```python
from build123d import *

# Parameters (mm, degrees)
F0_R     = 2
F1_DEPTH = 1
F2_R     = 0.99999


# Not quite as in the source:
# - a fillet or chamfer is up to 0.001 mm smaller than in the source, because OpenCascade refuses the exact size


with BuildPart() as f1:
    # F0 (on Top) → F1 (new body)
    with BuildSketch(Plane.XY):
        with BuildLine():
            Line((-56.070427214, 21.7097375971), (-58.2998616904, 23.7171294162))
            Line((-58.2998616904, 23.7171294162), (-61.9800800254, 19.6298328761))
            ThreePointArc((-61.9800800254, 19.6298328761), (-63.5129882811, 15.3010335004), (-61.5359947107, 11.156180285))
            Line((-61.5359947107, 11.156180285), (-35.2268663082, -12.5326653305))
            ThreePointArc((-35.2268663082, -12.5326653305), (-31.2120826701, -14.0737963776), (-27.1972990319, -12.5326653305))
            Line((-27.1972990319, -12.5326653305), (0, 11.9558927118))
            Line((0, 11.9558927118), (27.1972990319, -12.5326653305))
            ThreePointArc((27.1972990319, -12.5326653305), (31.2120826701, -14.0737963776), (35.2268663082, -12.5326653305))
            Line((35.2268663082, -12.5326653305), (61.5359947107, 11.156180285))
            ThreePointArc((61.5359947107, 11.156180285), (63.5129882811, 15.3010335004), (61.9800800254, 19.6298328761))
            Line((61.9800800254, 19.6298328761), (58.2998616904, 23.7171294162))
            Line((58.2998616904, 23.7171294162), (56.070427214, 21.7097375971))
            Line((56.070427214, 21.7097375971), (33.7760824497, 1.6358194063))
            Line((33.7760824497, 1.6358194063), (31.2120826701, -0.6728163648))
            Line((31.2120826701, -0.6728163648), (28.6480828904, 1.6358194063))
            Line((28.6480828904, 1.6358194063), (1.8948691733, 25.7245212353))
            Line((1.8948691733, 25.7245212353), (0, 27.4306691023))
            Line((0, 27.4306691023), (-1.8948691733, 25.7245212353))
            Line((-1.8948691733, 25.7245212353), (-28.6480828904, 1.6358194063))
            Line((-28.6480828904, 1.6358194063), (-31.2120826701, -0.6728163648))
            Line((-31.2120826701, -0.6728163648), (-33.7760824497, 1.6358194063))
            Line((-33.7760824497, 1.6358194063), (-56.070427214, 21.7097375971))
        make_face()
        with Locations((-31.2120826701, -8.0737963776)):
            Circle(F0_R, mode=Mode.SUBTRACT)
        Polygon((-53.6574585069, 9.4448453424), (-50.9809360815, 12.4174246443), (-35.0758352357, -1.9035924822), (-37.7523576611, -4.8761717841), align=None, mode=Mode.SUBTRACT)
        Polygon((-6.0931870421, 11.8520933749), (-22.4423732026, -2.868779965), (-25.118895628, 0.1037993369), (-8.7697094675, 14.8246726768), align=None, mode=Mode.SUBTRACT)
        with Locations((31.2120826701, -8.0737963776)):
            Circle(F0_R, mode=Mode.SUBTRACT)
        Polygon((22.4423732026, -2.868779965), (6.0931870421, 11.8520933749), (8.7697094675, 14.8246726768), (25.118895628, 0.1037993369), align=None, mode=Mode.SUBTRACT)
        Polygon((37.7523576611, -4.8761717841), (35.0758352357, -1.9035924822), (51.0113683193, 12.4448259544), (53.6878907447, 9.4722466525), align=None, mode=Mode.SUBTRACT)
        with Locations((-57.5212110725, 15.6150492379)):
            Circle(F0_R, mode=Mode.SUBTRACT)
        with Locations((0, 20.0296890894)):
            Circle(F0_R, mode=Mode.SUBTRACT)
        with Locations((57.5516433104, 15.6424505479)):
            Circle(F0_R, mode=Mode.SUBTRACT)
        Polygon((-55.7358619108, 22.0813100098), (-57.9652963872, 24.0887018289), (-58.2998616904, 23.7171294162), (-56.070427214, 21.7097375971), align=None)
        Polygon((-57.6307310841, 24.4602742417), (-57.9652963872, 24.0887018289), (-55.7358619108, 22.0813100098), (-55.4012966076, 22.4528824226), align=None)
        with BuildLine():
            Line((-53.9505127491, 28.5475707818), (-57.6307310841, 24.4602742417))
            Line((-57.6307310841, 24.4602742417), (-55.4012966076, 22.4528824226))
            Line((-55.4012966076, 22.4528824226), (-33.1069518433, 2.3789642318))
            Line((-33.1069518433, 2.3789642318), (-31.2120826701, 0.6728163648))
            Line((-31.2120826701, 0.6728163648), (-29.3172134968, 2.3789642318))
            Line((-29.3172134968, 2.3789642318), (-2.5639997796, 26.4676660607))
            Line((-2.5639997796, 26.4676660607), (0, 28.7763018319))
            Line((0, 28.7763018319), (2.5639997796, 26.4676660607))
            Line((2.5639997796, 26.4676660607), (29.3172134968, 2.3789642318))
            Line((29.3172134968, 2.3789642318), (31.2120826701, 0.6728163648))
            Line((31.2120826701, 0.6728163648), (33.1069518433, 2.3789642318))
            Line((33.1069518433, 2.3789642318), (55.4012966076, 22.4528824226))
            Line((55.4012966076, 22.4528824226), (57.6307310841, 24.4602742417))
            Line((57.6307310841, 24.4602742417), (53.9505127491, 28.5475707818))
            ThreePointArc((53.9505127491, 28.5475707818), (49.8056595337, 30.5245643522), (45.4768601581, 28.9916560965))
            Line((45.4768601581, 28.9916560965), (31.2120826701, 16.1475927553))
            Line((31.2120826701, 16.1475927553), (4.0147836382, 40.6361507976))
            ThreePointArc((4.0147836382, 40.6361507976), (0, 42.1772818447), (-4.0147836382, 40.6361507976))
            Line((-4.0147836382, 40.6361507976), (-31.2120826701, 16.1475927553))
            Line((-31.2120826701, 16.1475927553), (-45.4768601581, 28.9916560965))
            ThreePointArc((-45.4768601581, 28.9916560965), (-49.8056595337, 30.5245643522), (-53.9505127491, 28.5475707818))
        make_face()
        with Locations((-31.2120826701, 8.0737963776)):
            Circle(F0_R, mode=Mode.SUBTRACT)
        with Locations((31.2120826701, 8.0737963776)):
            Circle(F0_R, mode=Mode.SUBTRACT)
        Polygon((-46.3710360561, 19.0317138545), (-43.6945136306, 22.0042931564), (-34.3115040691, 13.5557933995), (-37.0313460748, 10.6222192229), align=None, mode=Mode.SUBTRACT)
        with Locations((-49.4916437962, 24.5327871436)):
            Circle(F0_R, mode=Mode.SUBTRACT)
        Polygon((-22.4423732026, 13.2788127903), (-25.118895628, 16.2513920922), (-8.7697094675, 30.9722654321), (-6.0931870421, 27.9996861302), align=None, mode=Mode.SUBTRACT)
        Polygon((6.0931870421, 27.9996861302), (8.7697094675, 30.9722654321), (25.118895628, 16.2513920922), (22.4423732026, 13.2788127903), align=None, mode=Mode.SUBTRACT)
        Polygon((37.0092128356, 10.6022903648), (34.3326904102, 13.5748696667), (43.6361429708, 21.9517359782), (46.3126653962, 18.9791566763), align=None, mode=Mode.SUBTRACT)
        with Locations((49.4332731364, 24.4802299654)):
            Circle(F0_R, mode=Mode.SUBTRACT)
        with Locations((0, 36.1772818447)):
            Circle(F0_R, mode=Mode.SUBTRACT)
        Polygon((-31.2120826701, 0), (-33.4415171465, 2.0073918191), (-33.7760824497, 1.6358194063), (-31.2120826701, -0.6728163648), (-28.6480828904, 1.6358194063), (-28.9826481936, 2.0073918191), align=None)
        Polygon((-33.1069518433, 2.3789642318), (-33.4415171465, 2.0073918191), (-31.2120826701, 0), (-28.9826481936, 2.0073918191), (-29.3172134968, 2.3789642318), (-31.2120826701, 0.6728163648), align=None)
        Polygon((0, 28.1034854671), (-2.2294344764, 26.096093648), (-1.8948691733, 25.7245212353), (0, 27.4306691023), (1.8948691733, 25.7245212353), (2.2294344764, 26.096093648), align=None)
        Polygon((-2.5639997796, 26.4676660607), (-2.2294344764, 26.096093648), (0, 28.1034854671), (2.2294344764, 26.096093648), (2.5639997796, 26.4676660607), (0, 28.7763018319), align=None)
        Polygon((31.2120826701, 0), (28.9826481936, 2.0073918191), (28.6480828904, 1.6358194063), (31.2120826701, -0.6728163648), (33.7760824497, 1.6358194063), (33.4415171465, 2.0073918191), align=None)
        Polygon((29.3172134968, 2.3789642318), (28.9826481936, 2.0073918191), (31.2120826701, 0), (33.4415171465, 2.0073918191), (33.1069518433, 2.3789642318), (31.2120826701, 0.6728163648), align=None)
        Polygon((57.9652963872, 24.0887018289), (55.7358619108, 22.0813100098), (56.070427214, 21.7097375971), (58.2998616904, 23.7171294162), align=None)
        Polygon((57.9652963872, 24.0887018289), (57.6307310841, 24.4602742417), (55.4012966076, 22.4528824226), (55.7358619108, 22.0813100098), align=None)
    extrude(amount=F1_DEPTH)

    # F2 (radius 1 in the source; OpenCascade refuses exactly that, so slightly less here)
    f2_edges = [f1.edges().sort_by_distance(p)[0] for p in [
        (-63.512988, 15.301034, 1),
        (-48.381431, -0.688243, 1),
        (-31.212083, -14.073796, 1),
        (-13.59865, -0.288386, 1),
        (13.59865, -0.288386, 1),
        (31.212083, -14.073796, 1),
        (48.381431, -0.688243, 1),
        (63.512988, 15.301034, 1),
        (57.965296, 24.088702, 1),
        (49.80566, 30.524564, 1),
        (38.344471, 22.569624, 1),
        (17.613433, 28.391872, 1),
        (0, 42.177282, 1),
        (-17.613433, 28.391872, 1),
        (-38.344471, 22.569624, 1),
        (-49.80566, 30.524564, 1),
        (-57.965296, 24.088702, 1),
    ]]
    fillet(f2_edges, radius=F2_R)


solid = f1.part
```
Input: part model. Units: mm. Frame: model coordinates. Coordinates: 2 decimals unless noted, no trailing zeros. Put each result on its own line as item: value. Start each with the question number.
1) Mould query, pull axis Y, two halves, no side actions, for faces 1 (the face through (-51.08, 23.32, 0.49)), 2 (the face through (-45.59, 2.18, 0.49)), 3 (the face through (48.375, -0.311, 0.699)). Classes: pulls with the +Y half, pulls with the -Y half, needs draft (parallel to the pull), parting line crosses it, or undercut.
2) Contact query for a flat-ended pin moving along its axis: pin 1 (2.5 mm diameter, centred on x = 57.55, y = 15.64, fed in from -Z). Output: stop coordinate, or through.
3) Ray query, L1, parallel to Y at x = 51, z = 0.4; L2, parallel to Y at x = 29.5, z = 0.45; L3, parallel to Y at x = 35, z = 0.15. Return the intervals inside material, ascending.
4) Cut plane A-A (x = 11.5). State how many separate pieces and enclosed holes the cut face has, plus the area to 3 significant figures.
Resolved:
1. face 1: undercut
1. face 2: undercut
1. face 3: pulls with the -Y half
2. pin 1: passes through
3. L1: y = 1.78 to 7.05, 12.43 to 17.14, 18.49 to 23.24, 25.72 to 30.25
3. L2: y = -13.71 to -9.11, -7.04 to 7.04, 9.11 to 17.55
3. L3: y = -12.71 to 2.74, 4.08 to 12.83, 14.18 to 19.54
4. separate pieces: 4
4. enclosed holes: 0
4. area: 19.6 mm2
